```python
from build123d import *

# Parameters (mm, degrees)
F0_W     = 85.6928378344
F0_H     = 86.1391574144
F1_DEPTH = 25.4
F2_R     = 18.2584183748
F3_DEPTH = 162.2124761343
F4_DEPTH = 25.4


with BuildPart() as f1:
    # F0 (on Front) → F1 (new body)
    with BuildSketch(Plane.XZ):
        with Locations((-7.4506e-06, 4.8927590251)):
            Rectangle(F0_W, F0_H)
    extrude(amount=F1_DEPTH)

    # F2 (on Front) → F3 (cut)
    with BuildSketch(Plane.XZ):
        Circle(F2_R)
    extrude(amount=F3_DEPTH, mode=Mode.SUBTRACT)

    # F4 (add): a face of the model
    f4_faces = [f1.faces().sort_by_distance(p)[0] for p in [
        (-7.4506e-06, -25.4, 46.747297943),
    ]]
    extrude(f4_faces, amount=F4_DEPTH)


solid = f1.part
```
Verification items for the finished model (mm, model axes). Coordinates: 2 decimals unless noted, no trailing zeros. Order: outer loops, then holes, each group sorted by start corner. A loop starts at its lowest first (then second) coordinate and runs counter-clockwise, first axis right, second up. Notation, with made-up numbers: (-3, 30.25) -> (24, 30.25) arc R26 cw to (24, 50.25) -> close; hole circle Ø6 at (24, -4.75). An arc over 180 degrees is marked (long way). Put each result on its own line as item: value. Start each with the question number.
1) Cross-section at C-C (y = -14). Enter the section's corners in (x, z), plus the area to 3 significant figures.
2) Release check for a two-part mould opening along X. For faces 1 (the cylindrical face through (-14.49, -25.04, -11.11)), 2 (the flat face through (42.846, -25, 4)), 3 (the flat face through (-42.846, -25, 4)), 4 (the flat face through (-1, -25, 47.962)) record: pulls with the +X half, pulls with the -X half, needs draft (parallel to the pull), parting line crosses it, or undercut.
3) Material ranges on L1, parallel to Z at x = 0, y = -27; L2, parallel to X at y = -15, z = 0; L3, parallel to Z at x = 11, y = -11, recorded low to high.
4) Cross-section at A-A (x = 0). Enter the section's corners in (y, z), plus the area to 3 significant figures.
5) Cross-section at B-B (z = 0). Enter the section's corners in (x, y).
Geometry check:
1. outline: (-42.85, -38.18) -> (42.85, -38.18) -> (42.85, 47.96) -> (-42.85, 47.96) -> close; hole circle Ø36.52 at (0, 0)
1. area: 6,330 mm^2
2. face 1: undercut
2. face 2: pulls with the +X half
2. face 3: pulls with the -X half
2. face 4: needs draft
3. L1: z = -38.18 to -18.26, 18.26 to 47.96
3. L2: x = -42.85 to -18.26, 18.26 to 42.85
3. L3: z = -38.18 to -14.57, 14.57 to 47.96
4. outline: (-50.8, -38.18) -> (0, -38.18) -> (0, -18.26) -> (-50.8, -18.26) -> close; (-50.8, 18.26) -> (0, 18.26) -> (0, 47.96) -> (-50.8, 47.96) -> close
4. area: 2,520 mm^2
5. outline: (-42.85, -50.8) -> (-18.26, -50.8) -> (-18.26, 0) -> (-42.85, 0) -> close; (18.26, -50.8) -> (42.85, -50.8) -> (42.85, 0) -> (18.26, 0) -> close
